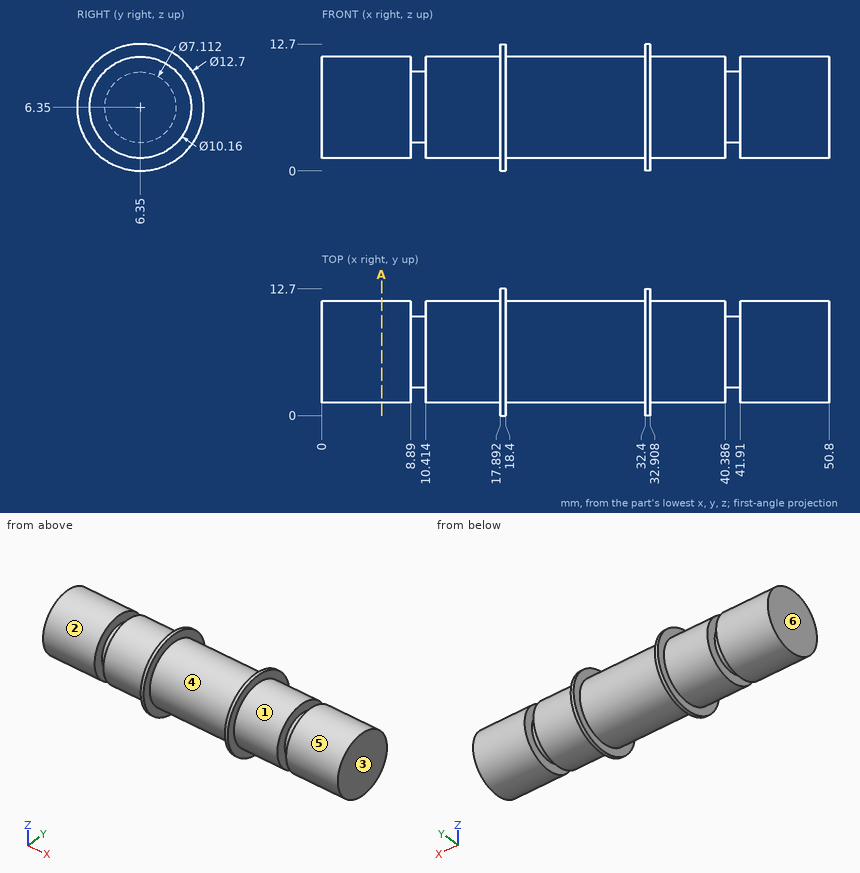
Can you work these out from the drawing? Everything is in mm from the part's minimum corner. A direction names the side the tool comes from. Give positions to 0.01 mm unless a question says otherwise; leave off trailing zeros. Loops run counter-clockwise (first coordinate to the right, second up) from the corner with the lowest first, then second, coordinate; pieces in that order, holes last. Notation, with made-up numbers: (-8.75, -22) - (10.25, -22) arc R19 ccw to (10.25, -8) - close; hole circle Ø11 at (-28, 16.5). An arc over 180 degrees is marked (long way). Answer as a JSON object with one key per item and string values.
Q1. If we mould it in two halves opening along X, with no side actions, what happens to the marked faces 3, 4, 5 and 6? For each: pulls with the +X half, pulls with the -X half, needs draft (parallel to the pull), parting line crosses it, or undercut.
Geometry says:
{"face 3": "pulls with the +X half", "face 4": "undercut", "face 5": "needs draft", "face 6": "pulls with the -X half"}
Q2. Will these pins go through, and if not, where does the flat tip stop? P1, Ø1.5, axis at x = 11, z = 2, coming from the -Y side; P2, Ø4, axis at x = 17.5, y = 10, coming from the -Z side; P3, Ø6, axis at x = 22, y = 1.5, coming from the -Z side.
Geometry says:
{"P1": "y = 2.77", "P2": "z = 0.23", "P3": "z = 1.62"}
Q3. Imagine slicing it at A-A on x = 6. Write out the boundary of the cut face in (y, z), plus the area to 3 significant figures.
Geometry says:
{"outline": "circle Ø10.16 at (6.35, 6.35)", "area": "81.1 mm²"}
Q4. If I drill on L1, parallel to X at y = 2.75, z = 4.5; L2, parallel to X at y = 2, z = 2.25; L3, parallel to Y at x = 14.5, z = 8.25, over which ranges is the centre line in solid material (lowest first)?
Geometry says:
{"L1": "0 to 8.89, 10.41 to 40.39, 41.91 to 50.8", "L2": "17.89 to 18.4, 32.4 to 32.91", "L3": "1.64 to 11.06"}
Q5. Which directions (+Z, -Z, +X, -X, +Y, -Y) give clear straight access to the entire face, cutting with the end or side of a thin tool? Please do the marked faces 1 and 2.
Geometry says:
{"face 1": "+X", "face 2": "-X"}
